Input: dimensioned drawing with shaded views. Units: mm. Origin: part minimum x, y, z. A direction names the side the tool comes from. Coordinates: 2 decimals unless noted, no trailing zeros. Order: outer loops, then holes, each group sorted by start corner. A loop starts at its lowest first (then second) coordinate and runs counter-clockwise, first axis right, second up. Notation, with made-up numbers: (41.25, 60.5) - (90.25, 60.5) arc R14 cw to (90.25, 67.5) - close; hole circle Ø8 at (-33.75, 65.5). An arc over 180 degrees is marked (long way). One line per question, with ' | ' between items. Start each with the question number.
(1) Access query for the marked faces 4, 5, 6, 7 and 8. Directions: +Z, -Z, +X, -X, +Y, -Y. A direction counts if a zero-diameter tool reaches every point of the face in a straight line with its end or side. Return the directions, or none.
(2) Section A-A (y = 28). Return the cut outline in (x, z).
(3) Section D-D (z = 22.5). Return the cut outline in (x, y), then the cut area to 3 significant figures.
(4) Section B-B (y = 12.5). Return the cut outline in (x, z), then the cut area to 3 significant figures.
(5) Contact query for flat-ended pins moving along their axis: P1, Ø13, axis at y = 15.5, z = 9.5, coming from the +X side; P2, Ø4, axis at y = 5, z = 19.5, coming from the -X side; P3, Ø6.5, axis at x = 38.5, z = 20, coming from the -Y side; P4, Ø7, axis at y = 12.5, z = 15.58, coming from the -X side. Output: stop coordinate, or through.
(6) Line query: line 1 along X through (y, z) = (6.5, 29); line 2 along Z through (x, y) = (53.95, 12.5); line 3 along Y through (x, z) = (18.5, 16.5). Output: solid intervals per line, ascending.
(7) Draft query along Z for the marked faces 1, 2 and 3. Return one class per face: +Z half, -Z half, draft (parallel to the pull), parting line (faces both ways), or undercut.
(8) Section C-C (x = 54). Return the cut outline in (y, z).
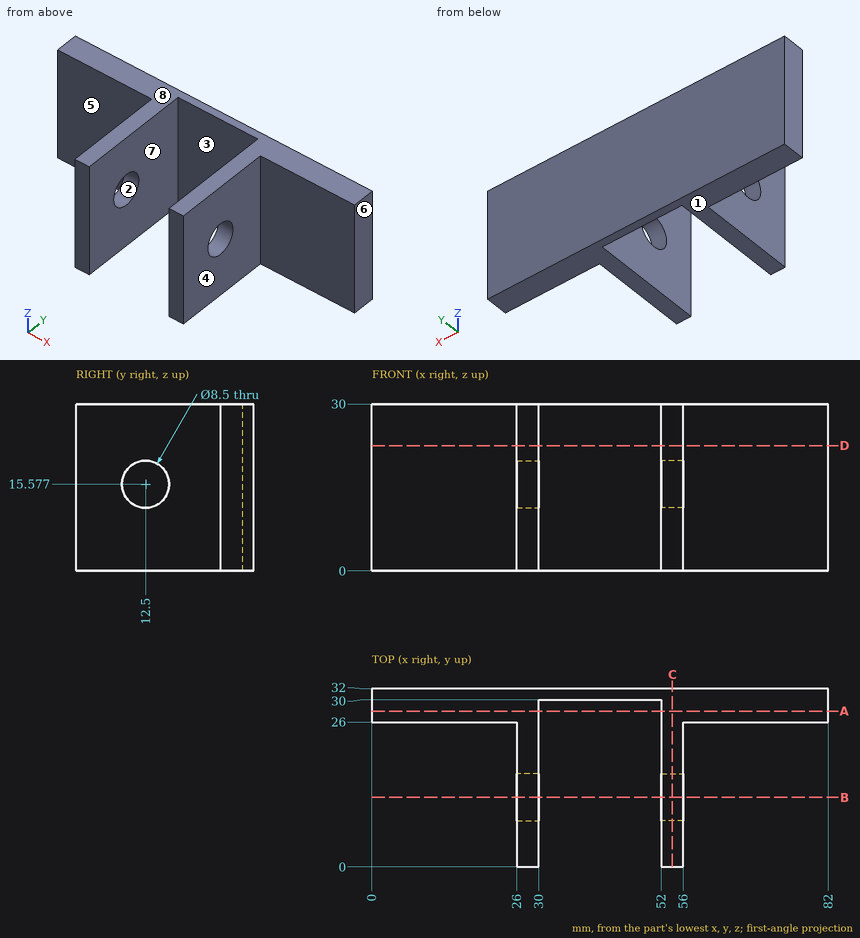
Response values:
1) face 4: +Z, -Z, +X, -Y | face 5: +Z, -Z, -X, -Y | face 6: +Z, -Z, +X, +Y, -Y | face 7: +Z, -Z, -Y | face 8: +Z, +X, -X, +Y, -Y
2) outline: (0, 0) - (30, 0) - (30, 30) - (0, 30) - close; (52, 0) - (82, 0) - (82, 30) - (52, 30) - close
3) outline: (0, 26) - (26, 26) - (26, 0) - (30, 0) - (30, 30) - (52, 30) - (52, 0) - (56, 0) - (56, 26) - (82, 26) - (82, 32) - (0, 32) - close | area: 612 mm²
4) outline: (26, 0) - (30, 0) - (30, 11.33) - (26, 11.33) - close; (26, 19.83) - (30, 19.83) - (30, 30) - (26, 30) - close; (52, 0) - (56, 0) - (56, 11.33) - (52, 11.33) - close; (52, 19.83) - (56, 19.83) - (56, 30) - (52, 30) - close | area: 172 mm²
5) P1: stops at x = 56 | P2: stops at x = 26 | P3: stops at y = 30 | P4: passes through
6) line 1: x = 26 to 30, 52 to 56 | line 2: z = 0 to 11.33, 19.83 to 30 | line 3: y = 26 to 32
7) face 1: -Z half | face 2: undercut | face 3: draft
8) outline: (0, 0) - (32, 0) - (32, 30) - (0, 30) - close; hole circle Ø8.5 at (12.5, 15.58)
